CAD build for the part. Positions are in the model's coordinates, mm. Give positions to 0.01 mm unless a question says otherwise; leave off trailing zeros. Write each loop counter-clockwise with the first axis right and the second up, starting at its lowest first coordinate (ties: lowest second). Pieces come first, ordered by that corner, then holes. Notation, with made-up numbers: M 31,21.5 L 47,21.5 A30 cw 47,51.5 Z; hole C 72,-16 d9. An arc over 180 degrees is marked long. One line per question, with ' | ' between items. Start each with the question number.
1. Wall check: L1, parallel to Y at x = 4.2, z = 2.5; L2, parallel to Z at x = 2.65, y = 38.5; L3, parallel to Z at x = 3.65, y = 34. Give the ranges that are in metal, low to high.
2. Cut at D-D, the plane z = 10. Write the cut outline in (x, y), then the cut area to 3 significant figures.
3. Cut at A-A, the plane x = 1.65. Write the cut outline in (y, z).
4. Cut at C-C, the plane y = 18. Write the cut outline in (x, z), then the cut area to 3 significant figures.
5. Flat gauge pins, fed straight in: pin 1 (1 mm diameter, centred on x = 2, y = -0.5, fed in from +Z); pin 2 (3 mm diameter, centred on x = 3.5, y = 0, fed in from +Z); pin 3 (2 mm diameter, centred on x = 3.5, y = -0.5, fed in from -Z). Where does each tip first touch, or does it go through?
6. Cut at B-B, the plane y = 36. Write the cut outline in (x, z), then the cut area to 3 significant figures.
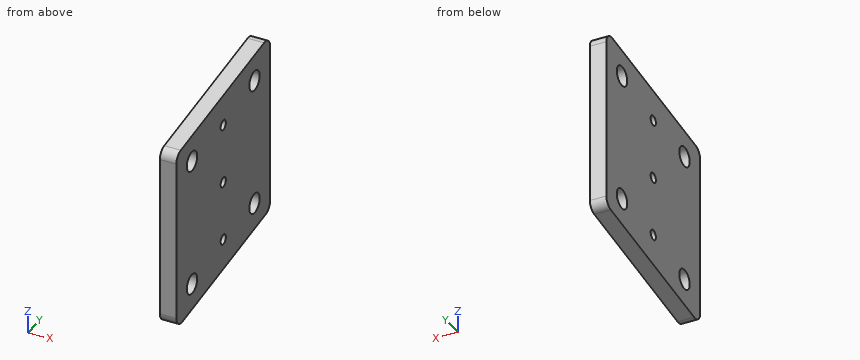
```python
from build123d import *

# Parameters (mm, degrees)
SKETCH1_R           = 3
SKETCH1_R_2         = 1.5
BOSS_EXTRUDE1_DEPTH = 5
FILLET1_R           = 3


with BuildPart() as part:
    # Sketch1 → Boss-Extrude1 (new body)
    with BuildSketch(Plane(origin=(0, 0, 0), x_dir=(0, 0, -1), z_dir=(1, 0, 0))):
        Polygon((-6.573014531, -9), (48.100102262, -9), (39.547342484, 45), (-15.125774308, 45), align=None)
        Circle(SKETCH1_R, mode=Mode.SUBTRACT)
        with Locations((38.676167805, 0)):
            Circle(SKETCH1_R, mode=Mode.SUBTRACT)
        with Locations((-5.701839852, 36)):
            Circle(SKETCH1_R, mode=Mode.SUBTRACT)
        with Locations((32.974327953, 36)):
            Circle(SKETCH1_R, mode=Mode.SUBTRACT)
        with Locations((16.487163977, 18)):
            Circle(SKETCH1_R_2, mode=Mode.SUBTRACT)
        with Locations((-1.512836023, 18)):
            Circle(SKETCH1_R_2, mode=Mode.SUBTRACT)
        with Locations((34.487163977, 18)):
            Circle(SKETCH1_R_2, mode=Mode.SUBTRACT)
    extrude(amount=BOSS_EXTRUDE1_DEPTH)

    # Fillet1
    fillet1_edges = [part.edges().sort_by_distance(p)[0] for p in [
        (2.5, 45, 15.125774308),
        (2.5, 45, -39.547342484),
        (2.5, -9, -48.100102262),
        (2.5, -9, 6.573014531),
    ]]
    fillet(fillet1_edges, radius=FILLET1_R)


solid = part.part
```
Here are the results:
1) L1: -9 to -1.66, 1.66 to 16.87, 19.13 to 45 | L2: -40.58 to -34.63, -31.32 to 4.04, 7.36 to 14.1 | L3: -41.29 to -35.21, -30.74 to 3.47, 7.94 to 13.38
2) outline: M 0,12.64 L 5,12.64 L 5,45 L 0,45 Z | area: 162 mm^2
3) outline: M -9,-44.59 A3 ccw -5.53,-47.55 L 42.47,-39.95 A3 ccw 45,-36.99 L 45,11.61 A3 ccw 41.53,14.58 L -6.47,6.97 A3 ccw -9,4.01 Z; hole C 0,-38.68 d6; hole C 0,0 d6; hole C 18,-34.49 d3; hole C 18,-16.49 d3; hole C 18,1.51 d3; hole C 36,-32.97 d6; hole C 36,5.7 d6
4) outline: M 0,-43.82 L 5,-43.82 L 5,-35.99 L 0,-35.99 Z; M 0,-32.99 L 5,-32.99 L 5,-17.99 L 0,-17.99 Z; M 0,-14.99 L 5,-14.99 L 5,0.01 L 0,0.01 Z; M 0,3.01 L 5,3.01 L 5,10.85 L 0,10.85 Z | area: 228 mm^2
5) pin 1: z = 8 | pin 2: z = 8.24 | pin 3: z = -46.91
6) outline: M 0,-40.97 L 5,-40.97 L 5,-35.97 L 0,-35.97 Z; M 0,-29.97 L 5,-29.97 L 5,2.7 L 0,2.7 Z; M 0,8.7 L 5,8.7 L 5,13.7 L 0,13.7 Z | area: 213 mm^2
